Source: CAD feature listing. Evaluate the final solid. Frame: model axes, mm. Face numbers are marked on the shaded views. Round coordinates to 2 decimals unless told otherwise and drop trailing zeros. Order: outer loops, then holes, each group sorted by start corner. A loop starts at its lowest first (then second) coordinate and runs counter-clockwise, first axis right, second up. Notation, with made-up numbers: (-3.75, 29.5) - (46.25, 29.5) arc R13 ccw to (46.25, 43.5) - close; hole circle Ø6 at (37, 56.5). An arc over 180 degrees is marked (long way). Put each result on its own line as item: value. Start each with the question number.
1) Contact query for flat-ended pins moving along their axis: P1, Ø2, axis at y = 17, z = -0.5, coming from the -X side; P2, Ø4, axis at x = -18.5, y = 38.5, coming from the +Z side; P3, Ø1, axis at x = 41, z = -10, coming from the +Y side. Output: stop coordinate, or through.
2) Line query: probe 1 along Y at (x, z) = (0, 48); probe 2 along X at (y, z) = (-18.5, 8); probe 3 along Y at (x, z) = (-27, -45.5). Output: solid intervals per line, ascending. Write a range as [from, to].
3) Mould query, pull axis X, two halves, no side actions, for the marked faces 1 and 2. Classes: +X half, -X half, draft (parallel to the pull), parting line (faces both ways), or undercut.
4) Section A-A on z = -22.5. Output: boundary loops of the cut face in (x, y), then the cut area to 3 significant figures.
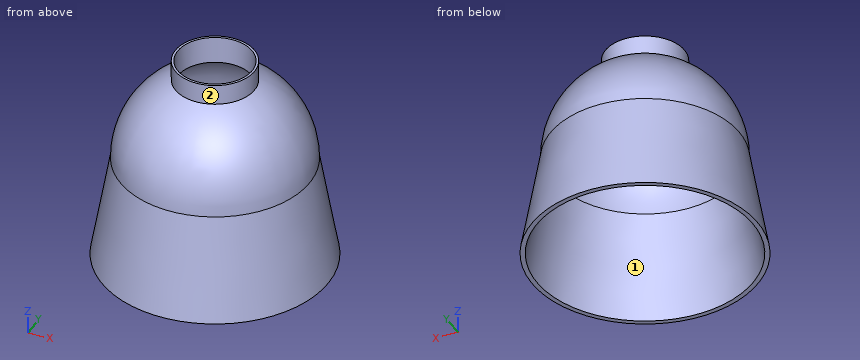
```python
from build123d import *

# Parameters (mm, degrees)
F2_R     = 21.2725
F2_R_2   = 20
F3_DEPTH = 57.15
F4_DEPTH = 57.151
F5_DEPTH = 42.545


with BuildPart() as f1:
    # F0 (on Front) → F1 (revolve)
    with BuildSketch(Plane.XZ):
        with BuildLine():
            Line((0, 48.26), (0, 50.8))
            ThreePointArc((0, 50.8), (-35.921024, 35.921024), (-50.8, 0))
            Line((-50.8, 0), (-48.26, 0))
            ThreePointArc((-48.26, 0), (-34.124973, 34.124973), (0, 48.26))
        make_face()
        Polygon((-48.26, 0), (-50.8, 0), (-60.723993, -56.281763), (-58.183993, -56.281763), align=None)
    revolve(axis=Axis((0, 0, -2.740882), (0, 0, -1)))

    # F2 (on Top) → F3 (join)
    with BuildSketch(Plane.XY):
        Circle(F2_R)
        Circle(F2_R_2, mode=Mode.SUBTRACT)
    extrude(amount=F3_DEPTH)

    # F2 (on Top) → F4 (cut, through all)
    with BuildSketch(Plane.XY):
        Circle(F2_R_2)
    extrude(amount=F4_DEPTH, mode=Mode.SUBTRACT)

    # F2 (on Top) → F5 (cut)
    with BuildSketch(Plane.XY):
        Circle(F2_R_2)
        Circle(F2_R)
        Circle(F2_R_2, mode=Mode.SUBTRACT)
    extrude(amount=F5_DEPTH, mode=Mode.SUBTRACT)


solid = f1.part
```
Answer sheet:
1. P1: x = -48.36
1. P2: z = 30.38
1. P3: y = 33.52
2. probe 1: [-21.27, -20], [20, 21.27]
2. probe 2: [-46.63, -43.85], [43.85, 46.63]
2. probe 3: [-52.26, -49.38], [49.38, 52.26]
3. face 1: undercut
3. face 2: parting line
4. outline: circle Ø109.53 at (0, 0); hole circle Ø104.45 at (0, 0)
4. area: 854 mm^2
